from build123d import *

# Parameters (mm, degrees)
SKETCH4_R            = 2.667
CUT_EXTRUDE2_DEPTH   = 2.921
M3_CLEARANCE_HOLE1_D = 3.2


with BuildPart() as part:
    # Sketch1 → Revolve1 (revolve)
    with BuildSketch(Plane(origin=(0, 0, 0), x_dir=(0, 0, -1), z_dir=(1, 0, 0))):
        Polygon((0, 5.3848), (9.9441, 5.3848), (9.9441, 3.3528), (4.7244, 3.3528), (4.7244, 0), (0, 0), align=None)
    revolve(axis=Axis((0, 0, 0), (0, 1, 0)))

    # Sketch4 → Cut-Extrude2 (cut)
    with BuildSketch(Plane.XZ):
        with Locations(Location((0, 0, 0), (0, 0, 270))):
            Circle(SKETCH4_R)
    extrude(amount=-CUT_EXTRUDE2_DEPTH, mode=Mode.SUBTRACT)

    # M3 Clearance Hole1 (through all)
    with Locations(Plane(origin=(0, 5.3848, 0), x_dir=(1, 0, 0), z_dir=(0, 1, 0))):
        with Locations((-6.985, 0), (0, 0), (6.985, 0), (0, 6.985), (0, -6.985)):
            Hole(M3_CLEARANCE_HOLE1_D / 2)


solid = part.part
Can you work these out from the model? Positions are in its coordinate system, mm. A direction names the side the tool comes from. Round coordinates to 2 decimals unless told otherwise and drop trailing zeros. Write each loop counter-clockwise with the first axis right and the second up, starting at its lowest first coordinate (ties: lowest second). Pieces come first, ordered by that corner, then holes. Notation, with made-up numbers: (78, 58.25) -> (116, 58.25) arc R25 ccw to (116, 97.25) -> close; hole circle Ø8 at (5.5, 72.25). An arc over 180 degrees is marked (long way). One line per question, with ' | ' between items. Start each with the question number.
1) Suppose I cut it at D-D on y = 4.95. Write out the boundary of the cut face in (x, z) (3 decimals), then the cut area to 3 significant figures.
2) I need wall thicknesses on line 1 (Z direction, x = 0, y = 4.05) (3 decimals); line 2 (Z direction, x = 0.5, y = 5.1); line 3 (Y direction, x = 3.5, z = -5.25). Which ranges of each line are inside material? Lowest first, please. Write a range as [from, to].
3) Suppose I cut it at B-B on z = 0. Write out the boundary of the cut face in (x, y) (3 decimals), then the cut area to 3 significant figures.
4) On a 3-axis mill with a long thin cutter (end or side, diameter ignored), from which of +Z, -Z, +X, -X, +Y, -Y can I reach the whole of each face in a straight line? I mean faces 4 (the cylindrical face through (0.21, 4.35, 5.4)), 5 (the cylindrical face through (-1.62, 1.44, 2.12)). Say none if no direction works.
5) If we mould it in two halves opening along Z, with no side actions, what happens to faces 1 (the flat face through (-2.3, 3.353, -4.3)), 2 (the cylindrical face through (0.347, 4.355, -5.423)), 3 (the cylindrical face through (-3.984, 1.653, -2.54))? For each: released by +Z, released by -Z, zero draft, split by the parting line, or undercut.
6) Suppose I cut it at C-C on x = 7.75. Write out the boundary of the cut face in (y, z), then the cut area to 3 significant figures.
7) I'm going to push flat-ended pins straight in: P1, Ø2, axis at y = 3, z = -3, coming from the +X side; P2, Ø3, axis at y = 2, z = -1, coming from the -X side; P3, Ø3, axis at x = -1, y = 2, coming from the +Z side. Where does each tip first touch, or does it pass through?
8) Suppose I cut it at A-A on x = 0. Write out the boundary of the cut face in (y, z) (3 decimals), then the cut area to 3 significant figures.
Return value:
1) outline: circle Ø19.888 at (0, 0); hole circle Ø3.2 at (-6.985, 0); hole circle Ø3.2 at (0, -6.985); hole circle Ø3.2 at (0, 0); hole circle Ø3.2 at (0, 6.985); hole circle Ø3.2 at (6.985, 0) | area: 270 mm2
2) line 1: z = [-9.944, -8.585], [-5.385, -1.6], [1.6, 5.385], [8.585, 9.944] | line 2: z = [-9.93, -8.5], [-5.47, -1.52], [1.52, 5.47], [8.5, 9.93] | line 3: y = [3.35, 5.38]
3) outline: (-9.944, 3.353) -> (-8.585, 3.353) -> (-8.585, 5.385) -> (-9.944, 5.385) -> close; (-5.385, 3.353) -> (-4.724, 3.353) -> (-4.724, 0) -> (-2.667, 0) -> (-2.667, 2.921) -> (-1.6, 2.921) -> (-1.6, 5.385) -> (-5.385, 5.385) -> close; (1.6, 2.921) -> (2.667, 2.921) -> (2.667, 0) -> (4.724, 0) -> (4.724, 3.353) -> (5.385, 3.353) -> (5.385, 5.385) -> (1.6, 5.385) -> close; (8.585, 3.353) -> (9.944, 3.353) -> (9.944, 5.385) -> (8.585, 5.385) -> close | area: 35.6 mm2
4) face 4: +Y, -Y | face 5: -Y
5) face 1: zero draft | face 2: undercut | face 3: split by the parting line
6) outline: (3.35, -6.23) -> (5.38, -6.23) -> (5.38, -1.41) -> (3.35, -1.41) -> close; (3.35, 1.41) -> (5.38, 1.41) -> (5.38, 6.23) -> (3.35, 6.23) -> close | area: 19.6 mm2
7) P1: stops at x = 9.73 | P2: stops at x = -9.94 | P3: stops at z = 9.94
8) outline: (0, -4.724) -> (3.353, -4.724) -> (3.353, -5.385) -> (5.385, -5.385) -> (5.385, -1.6) -> (2.921, -1.6) -> (2.921, -2.667) -> (0, -2.667) -> close; (0, 2.667) -> (2.921, 2.667) -> (2.921, 1.6) -> (5.385, 1.6) -> (5.385, 5.385) -> (3.353, 5.385) -> (3.353, 4.724) -> (0, 4.724) -> close; (3.353, -9.944) -> (5.385, -9.944) -> (5.385, -8.585) -> (3.353, -8.585) -> close; (3.353, 8.585) -> (5.385, 8.585) -> (5.385, 9.944) -> (3.353, 9.944) -> close | area: 35.6 mm2
